```python
from build123d import *

# Parameters (mm, degrees)
BRACKET_DEPTH       = 11.5
BOSS_EXTRUDE1_START = -3
BOSS_EXTRUDE1_DEPTH = 3
BOSS_EXTRUDE2_START = -3
SKETCH15_R          = 2
BOSS_EXTRUDE2_DEPTH = 3.5


with BuildPart() as part:
    # Sketch9 → Bracket (new body)
    with BuildSketch(Plane(origin=(0, 0, 0), x_dir=(1, 0, 0), z_dir=(0, 1, 0))):
        with BuildLine():
            Line((5.15, -5), (4.65, -5))
            Line((4.65, -5), (3.35, -5))
            Line((3.35, -5), (3.35, -7))
            Line((3.35, -7), (6.4, -7))
            ThreePointArc((6.4, -7), (6.930330086, -6.780330086), (7.15, -6.25))
            Line((7.15, -6.25), (7.15, -5))
            Line((7.15, -5), (7.15, -3.25))
            ThreePointArc((7.15, -3.25), (7.369669914, -2.719669914), (7.9, -2.5))
            Line((7.9, -2.5), (21.4, -2.5))
            ThreePointArc((21.4, -2.5), (21.930330086, -2.280330086), (22.15, -1.75))
            Line((22.15, -1.75), (22.15, 24.75))
            ThreePointArc((22.15, 24.75), (21.930330086, 25.280330086), (21.4, 25.5))
            Line((21.4, 25.5), (7.9, 25.5))
            ThreePointArc((7.9, 25.5), (7.369669914, 25.719669914), (7.15, 26.25))
            Line((7.15, 26.25), (7.15, 28))
            Line((7.15, 28), (7.15, 29.75))
            ThreePointArc((7.15, 29.75), (6.930330086, 30.280330086), (6.4, 30.5))
            Line((6.4, 30.5), (5.15, 30.5))
            Line((5.15, 30.5), (3.35, 30.5))
            Line((3.35, 30.5), (3.35, 28.5))
            Line((3.35, 28.5), (5.15, 28.5))
            Line((5.15, 28.5), (5.15, 28))
            Line((5.15, 28), (5.15, 23.5))
            Line((5.15, 23.5), (20.15, 23.5))
            Line((20.15, 23.5), (20.15, -0.5))
            Line((20.15, -0.5), (5.15, -0.5))
            Line((5.15, -0.5), (5.15, -5))
        make_face()
    extrude(amount=BRACKET_DEPTH)

    # Sketch12 → Boss-Extrude1 (add)
    with BuildSketch(Plane(origin=(0, 0, 0), x_dir=(1, 0, 0), z_dir=(0, 1, 0)).offset(BOSS_EXTRUDE1_START)):
        with BuildLine():
            Line((3.134136634, -6.799408153), (-15.169112008, 10.208954707))
            ThreePointArc((-15.169112008, 10.208954707), (-17.445237733, 24.907700028), (-3.6745965, 30.529381479))
            ThreePointArc((-3.6745965, 30.529381479), (-3.571695801, 30.507381696), (-3.466728879, 30.5))
            Line((-3.466728879, 30.5), (6.4, 30.5))
            ThreePointArc((6.4, 30.5), (6.930330086, 30.280330086), (7.15, 29.75))
            Line((7.15, 29.75), (7.15, 26.25))
            ThreePointArc((7.15, 26.25), (7.369669914, 25.719669914), (7.9, 25.5))
            Line((7.9, 25.5), (21.4, 25.5))
            ThreePointArc((21.4, 25.5), (21.930330086, 25.280330086), (22.15, 24.75))
            Line((22.15, 24.75), (22.15, -1.75))
            ThreePointArc((22.15, -1.75), (21.930330086, -2.280330086), (21.4, -2.5))
            Line((21.4, -2.5), (7.9, -2.5))
            ThreePointArc((7.9, -2.5), (7.369669914, -2.719669914), (7.15, -3.25))
            Line((7.15, -3.25), (7.15, -6.25))
            ThreePointArc((7.15, -6.25), (6.930330086, -6.780330086), (6.4, -7))
            Line((6.4, -7), (3.644676233, -7))
            ThreePointArc((3.644676233, -7), (3.370410043, -6.948053048), (3.134136634, -6.799408153))
        make_face()
    extrude(amount=BOSS_EXTRUDE1_DEPTH)

    # Sketch15 → Boss-Extrude2 (add)
    with BuildSketch(Plane(origin=(0, 0, 0), x_dir=(1, 0, 0), z_dir=(0, 1, 0)).offset(BOSS_EXTRUDE2_START)):
        with Locations(Location((-7, 26.071067812, 0), (0, 0, 270))):
            Circle(SKETCH15_R)
        with Locations(Location((0.071067812, 19, 0), (0, 0, 270))):
            Circle(SKETCH15_R)
        with Locations(Location((-7, 11.928932188, 0), (0, 0, 270))):
            Circle(SKETCH15_R)
        with Locations(Location((-14.071067812, 19, 0), (0, 0, 270))):
            Circle(SKETCH15_R)
    extrude(amount=-BOSS_EXTRUDE2_DEPTH)


solid = part.part
```
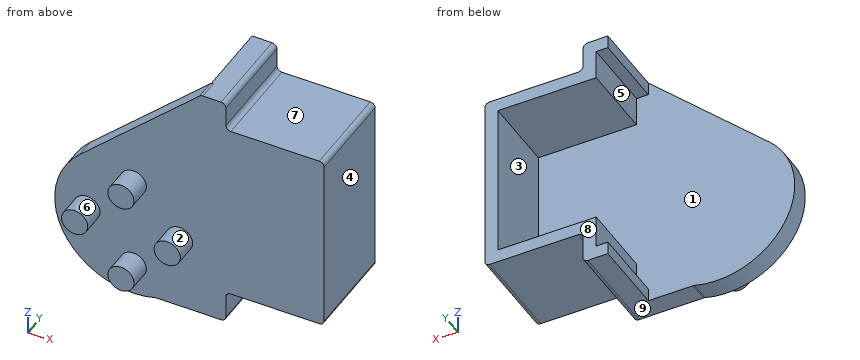
Here's how the part is built. I have some questions about the finished solid (model axes, mm). Face numbers are marked on the shaded views. A direction names the side the tool comes from. Coordinates: 2 decimals unless noted, no trailing zeros. Order: outer loops, then holes, each group sorted by start corner. A loop starts at its lowest first (then second) coordinate and runs counter-clockwise, first axis right, second up.
Item 1: If we section it at C-C, the plane y = 1.5: List the corners of the cut face in (x, z) for me.
Response values:
outline: (3.35, -30.5) - (6.4, -30.5) arc R0.75 ccw to (7.15, -29.75) - (7.15, -26.25) arc R0.75 cw to (7.9, -25.5) - (21.4, -25.5) arc R0.75 ccw to (22.15, -24.75) - (22.15, 1.75) arc R0.75 ccw to (21.4, 2.5) - (7.9, 2.5) arc R0.75 cw to (7.15, 3.25) - (7.15, 6.25) arc R0.75 ccw to (6.4, 7) - (3.35, 7) - (3.35, 5) - (5.15, 5) - (5.15, 0.5) - (20.15, 0.5) - (20.15, -23.5) - (5.15, -23.5) - (5.15, -28.5) - (3.35, -28.5) - close
Item 2: Which directions (+Z, -Z, +X, -X, +Y, -Y) give clear straight access to the entire face, cutting with the end or side of a thin tool? Please do the marked faces 5, 6, 7, 8 and 9.
Response values:
face 5: -X, +Y
face 6: -Y
face 7: +Z, +X, +Y, -Y
face 8: +Z, -Z, +X, -X, +Y
face 9: -Z, +X, +Y, -Y
Item 3: Thinking about a two-plate mould opening in Z: for the marked faces 1, 2, 3 and 4, which applies, pulls with the +Z half, pulls with the -Z half, needs draft (parallel to the pull), parting line crosses it, or undercut?
Response values:
face 1: undercut
face 2: parting line crosses it
face 3: undercut
face 4: needs draft
Item 4: If we section it at B-B, the plane z = -19: List the corners of the cut face in (x, y) for me, then the cut area to 3 significant figures.
Response values:
outline: (-19, -3) - (-16.07, -3) - (-16.07, -6.5) - (-12.07, -6.5) - (-12.07, -3) - (-1.93, -3) - (-1.93, -6.5) - (2.07, -6.5) - (2.07, -3) - (22.15, -3) - (22.15, 11.5) - (20.15, 11.5) - (20.15, 0) - (-19, 0) - close
area: 174 mm2
Item 5: If we section it at D-D, the plane y = -5: List the corners of the cut face in (x, z) for me.
Response values:
outline: circle Ø4 at (-14.07, -19); circle Ø4 at (-7, -26.07); circle Ø4 at (-7, -11.93); circle Ø4 at (0.07, -19)
Item 6: If we section it at A-A, the plane x = 17.5: List the corners of the cut face in (y, z) for me.
Response values:
outline: (-3, -25.5) - (11.5, -25.5) - (11.5, -23.5) - (0, -23.5) - (0, 0.5) - (11.5, 0.5) - (11.5, 2.5) - (-3, 2.5) - close
Item 7: I need wall thicknesses on probe 1 along Z at (x, y) = (15, 5.75); probe 2 along Z at (x, y) = (4, 9.5); probe 3 along X at (y, z) = (1.25, 4). Which ranges of each line are inside material? Lowest first, please.
Response values:
probe 1: z = -25.5 to -23.5, 0.5 to 2.5
probe 2: z = -30.5 to -28.5, 5 to 7
probe 3: x = 5.15 to 7.15
Item 8: I'm going to push flat-ended pins straight in: pin 1 Ø8 at (x, z) = (-15, -24.5) entering from +Y; pin 2 Ø1.6 at (y, z) = (5, 5.5) entering from -X; pin 3 Ø4 at (x, y) = (12, 2) entering from -Z. Where does each tip first touch, or does it pass through?
Response values:
pin 1: stops at y = 0
pin 2: stops at x = 3.35
pin 3: stops at z = -25.5
